from build123d import *

# Parameters (mm, degrees)
BOSS_EXTRUDE1_DEPTH = 1.5875
SKETCH2_W           = 36.068
SKETCH2_H           = 1.5875
BOSS_EXTRUDE2_DEPTH = 21.2725
SKETCH3_W           = 1.5875
SKETCH3_H           = 25.654
BOSS_EXTRUDE3_DEPTH = 6.35
HOLE1_D             = 5.08
HOLE1_DEPTH         = 15.875
SKETCH9_W           = 48.514
SKETCH9_H           = 25.908
BOSS_EXTRUDE4_DEPTH = 30.988
SKETCH11_W          = 80.424320956
SKETCH11_H          = 56.498512817
BOSS_EXTRUDE5_DEPTH = 1.5875


with BuildPart() as part:
    # Sketch1 → Boss-Extrude1 (new body)
    with BuildSketch(Plane(origin=(0, 0, 0), x_dir=(1, 0, 0), z_dir=(0, 1, 0))):
        Polygon((0, 0), (0, -25.4), (13.2588, -56.388), (31.9532, -56.388), (31.9532, -49.3268), (80.4672, -49.3268), (80.4672, 0), align=None)
    extrude(amount=BOSS_EXTRUDE1_DEPTH)

    # Sketch2 → Boss-Extrude2 (add)
    with BuildSketch(Plane.XZ):
        with Locations((18.034, 0.79375)):
            Rectangle(SKETCH2_W, SKETCH2_H)
    extrude(amount=BOSS_EXTRUDE2_DEPTH)

    # Sketch3 → Boss-Extrude3 (add)
    with BuildSketch(Plane.XY.offset(1.5875)):
        with Locations((35.27425, -21.971)):
            Rectangle(SKETCH3_W, SKETCH3_H)
        with Locations((0.79375, -21.971)):
            Rectangle(SKETCH3_W, SKETCH3_H)
    extrude(amount=BOSS_EXTRUDE3_DEPTH)

    # Hole1
    with Locations(Plane(origin=(0, 0, 0), x_dir=(-1, 0, 0), z_dir=(0, 0, -1))):
        with Locations((-18.034, -9.8425)):
            Hole(HOLE1_D / 2, depth=HOLE1_DEPTH)

    # Sketch9 → Boss-Extrude4 (add)
    with BuildSketch(Plane(origin=(0, 1.5875, 0), x_dir=(1, 0, 0), z_dir=(0, 1, 0))):
        with Locations((46.863, -25.7048)):
            Rectangle(SKETCH9_W, SKETCH9_H)
    extrude(amount=BOSS_EXTRUDE4_DEPTH)

    # Sketch11 → Boss-Extrude5 (add)
    with BuildSketch(Plane(origin=(0, 1.5875, 0), x_dir=(1, 0, 0), z_dir=(0, 1, 0))):
        with Locations((40.212160478, -28.249256409)):
            Rectangle(SKETCH11_W, SKETCH11_H)
    extrude(amount=-BOSS_EXTRUDE5_DEPTH)


solid = part.part
Work out the finished part from the listing and answer in its coordinate system (mm). A direction names the side the tool comes from. Coordinates: 2 decimals unless noted, no trailing zeros. Loops run counter-clockwise (first coordinate to the right, second up) from the corner with the lowest first, then second, coordinate; pieces in that order, holes last. Notation, with made-up numbers: M -36,50.5 L 0,50.5 A20 cw 0,75.5 Z; hole C -23,73 d4. An arc over 180 degrees is marked long. Answer in a Markdown table with one row per item. Add a question column.
1. Find section A-A, the plane y = -28.5. Write down the section's boundary in (x, z).
2. Find section B-B, the plane x = 29.5. Write down the section's boundary in (y, z).
3. A tool of negligible diameter and unlimited length cuts with its end or side. For faces 5 (the flat face through (36.068, -18, 4)), 6 (the flat face through (71.12, 17, 26)), 7 (the flat face through (47, 17, 12.751)), from which of +Z, -Z, +X, -X, +Y, -Y can it reach the whole face along a straight path? Write none if from no direction.
4. Consider L1, parallel to Z at x = 39, y = 17; L2, parallel to Z at x = 25, y = -9.5. Determine where each line is inside the solid, lowest interval first.
5. Find section D-D, the plane y = 17.5. Write down the section's boundary in (x, z).
6. Find section C-C, the plane z = 14. Write down the section's boundary in (x, y).
7. The mould has two halves that part along X. Classify faces 1 (the flat face through (40, 0, 28)), 2 (the flat face through (34.48, -22, 5)), 3 (the flat face through (18, -13, 1.588)), 4 (the flat face through (22.606, 17, 26)): pulls with the +X half, pulls with the -X half, needs draft (parallel to the pull), parting line crosses it, or undercut.
8. Flat-ended cylindrical pins translate along their axes: P1, Ø1.9, axis at y = -21.5, z = 6, coming from the -X side; P2, Ø0.8, axis at x = 0.5, y = -20.5, coming from the +Z side; P3, Ø1.7, axis at y = 0.5, z = 51.5, coming from the +X side; P4, Ø20.5, axis at y = 12, z = 32, coming from the -X side. Find the tip coordinate at first contact, or state that the pin passes through.
Reported:
| question | item | result |
|---|---|---|
| 1 | outline | M 0,1.59 L 1.59,1.59 L 1.59,7.94 L 0,7.94 Z; M 34.48,1.59 L 36.07,1.59 L 36.07,7.94 L 34.48,7.94 Z |
| 2 | outline | M -21.27,0 L 1.59,0 L 1.59,12.75 L 32.58,12.75 L 32.58,38.66 L 1.59,38.66 L 1.59,56.5 L 0,56.5 L 0,1.59 L -21.27,1.59 Z |
| 3 | face 5 | +Z, -Z, +X, -Y |
| 3 | face 6 | +Z, -Z, +X, +Y |
| 3 | face 7 | -Z, +X, -X, +Y |
| 4 | L1 | z = 12.75 to 38.66 |
| 4 | L2 | z = 0 to 1.59 |
| 5 | outline | M 22.61,12.75 L 71.12,12.75 L 71.12,38.66 L 22.61,38.66 Z |
| 6 | outline | M 0,0 L 80.47,0 L 80.47,1.59 L 71.12,1.59 L 71.12,32.58 L 22.61,32.58 L 22.61,1.59 L 0,1.59 Z |
| 7 | face 1 | needs draft |
| 7 | face 2 | undercut |
| 7 | face 3 | undercut |
| 7 | face 4 | pulls with the -X half |
| 8 | P1 | stops at x = 0 |
| 8 | P2 | stops at z = 7.94 |
| 8 | P3 | stops at x = 80.42 |
| 8 | P4 | stops at x = 22.61 |
